```python
from build123d import *

# Parameters (mm, degrees)
SKETCH1_W           = 20
SKETCH1_H           = 14
SKETCH1_W_2         = 16
SKETCH1_H_2         = 10
BOSS_EXTRUDE1_DEPTH = 100
SKETCH2_W           = 50
SKETCH2_H           = 30
BOSS_EXTRUDE2_DEPTH = 2
SKETCH3_R           = 2.5
CUT_EXTRUDE1_DEPTH  = 2
SKETCH4_R           = 2.5
CUT_EXTRUDE2_DEPTH  = 106.399240984
FILLET1_R           = 1


with BuildPart() as part:
    # Sketch1 → Boss-Extrude1 (new body)
    with BuildSketch(Plane(origin=(0, 0, 0), x_dir=(1, 0, 0), z_dir=(0, 1, 0))):
        Rectangle(SKETCH1_W, SKETCH1_H)
        Rectangle(SKETCH1_W_2, SKETCH1_H_2, mode=Mode.SUBTRACT)
    extrude(amount=BOSS_EXTRUDE1_DEPTH)

    # Sketch2 → Boss-Extrude2 (add)
    with BuildSketch(Plane(origin=(0, 0, 0), x_dir=(-1, 0, 0), z_dir=(0, -1, 0))):
        Rectangle(SKETCH2_W, SKETCH2_H)
    extrude(amount=BOSS_EXTRUDE2_DEPTH)

    # Sketch3 → Cut-Extrude1 (cut)
    with BuildSketch(Plane(origin=(0, 0, 0), x_dir=(1, 0, 0), z_dir=(0, 1, 0))):
        with Locations(Location((18, -8, 0), (0, 0, 270))):
            Circle(SKETCH3_R)
        with Locations(Location((18, 8, 0), (0, 0, 90))):
            Circle(SKETCH3_R)
        with Locations(Location((-18, -8, 0), (0, 0, 90))):
            Circle(SKETCH3_R)
        with Locations(Location((-18, 8, 0), (0, 0, 270))):
            Circle(SKETCH3_R)
    extrude(amount=-CUT_EXTRUDE1_DEPTH, mode=Mode.SUBTRACT)

    # Sketch4 → Cut-Extrude2 (cut, through all)
    with BuildSketch(Plane.XY.offset(7)):
        with Locations((0, 87)):
            Circle(SKETCH4_R)
    extrude(amount=-CUT_EXTRUDE2_DEPTH, mode=Mode.SUBTRACT)

    # Fillet1
    fillet1_edges = [part.edges().sort_by_distance(p)[0] for p in [
        (-10, 100, 0),
        (0, 100, 7),
        (10, 100, 0),
        (0, 0, 7),
        (-10, 0, 0),
        (0, 0, -7),
        (10, 0, 0),
        (10, 50, 7),
        (-10, 50, 7),
        (-10, 50, -7),
        (10, 50, -7),
        (0, 100, -7),
    ]]
    fillet(fillet1_edges, radius=FILLET1_R)


solid = part.part
```
Model file for the job. Use its own axes, mm. A direction names the side the tool comes from. Give positions to 0.01 mm unless a question says otherwise; leave off trailing zeros. Order: outer loops, then holes, each group sorted by start corner. A loop starts at its lowest first (then second) coordinate and runs counter-clockwise, first axis right, second up.
1) Pin check, flat tips, straight feed: pin 1 (5 mm diameter, centred on y = 67.5, z = -2, fed in from +X); pin 2 (8 mm diameter, centred on y = 62.5, z = -0.5, fed in from -X); pin 3 (20 mm diameter, centred on x = -0.5, y = 67, fed in from +Z); pin 4 (4.5 mm diameter, centred on x = 18, z = -8, fed in from -Y). Stop position of each tip, or through.
2) Wall check: probe 1 along X at (y, z) = (-1.2, -8); probe 2 along X at (y, z) = (71, 1.75); probe 3 along Z at (x, y) = (-0.5, 38.5). Give the ranges that are in metal, low to high.
3) Saw through at B-B, the plane x = -18. Write the cut outline in (y, z).
4) 3-axis set-ups, long thin cutter, end or side, ignore diameter. For faces 1 (the flat face through (10, 49, 0)), 2 (the flat face through (0, -2, 0)), 3 (the flat face through (0, 0, -10)), 4 (the flat face through (0, 49, -7)): which of +Z, -Z, +X, -X, +Y, -Y reach the whole face in a straight line?
5) Saw through at C-C, the plane y = 36. Write the cut outline in (x, z).
6) Saw through at D-D, the plane z = -2.5. Write the cut outline in (x, y), then the cut area to 3 significant figures.
7) Mould opens along X. For faces 5 (the flat face through (-10, 49, 0)), 6 (the flat face through (0, -1, -15)), 7 (the cylindrical face through (20.11, -0.99, 9.34)), 8 (the flat face through (25, -1, 0)) say: +X half, -X half, draft (parallel to the pull), parting line (faces both ways), or undercut.
8) Saw through at A-A, the plane y = 87. Write the cut outline in (x, z), then the cut area to 3 significant figures.
Computed:
1. pin 1: stops at x = 10
1. pin 2: stops at x = -10
1. pin 3: stops at z = 7
1. pin 4: passes through
2. probe 1: x = -25 to -20.5, -15.5 to 15.5, 20.5 to 25
2. probe 2: x = -10 to -8, 8 to 10
2. probe 3: z = -7 to -5, 5 to 7
3. outline: (-2, -15) - (0, -15) - (0, -10.5) - (-2, -10.5) - close; (-2, -5.5) - (0, -5.5) - (0, 5.5) - (-2, 5.5) - close; (-2, 10.5) - (0, 10.5) - (0, 15) - (-2, 15) - close
4. face 1: +Z, -Z, +X, +Y
4. face 2: +Z, -Z, +X, -X, -Y
4. face 3: +Y
4. face 4: -Z, +X, -X, +Y
5. outline: (-10, -6) arc R1 ccw to (-9, -7) - (9, -7) arc R1 ccw to (10, -6) - (10, 6) arc R1 ccw to (9, 7) - (-9, 7) arc R1 ccw to (-10, 6) - close; hole (-8, -5) - (8, -5) - (8, 5) - (-8, 5) - close
6. outline: (-25, -2) - (25, -2) - (25, 0) - (11, 0) arc R1 cw to (10, 1) - (10, 99) arc R1 ccw to (9, 100) - (8, 100) - (8, 0) - (-8, 0) - (-8, 100) - (-9, 100) arc R1 ccw to (-10, 99) - (-10, 1) arc R1 cw to (-11, 0) - (-25, 0) - close
6. area: 500 mm2
7. face 5: -X half
7. face 6: draft
7. face 7: undercut
7. face 8: +X half
8. outline: (-10, -6) arc R1 ccw to (-9, -7) - (-2.5, -7) - (-2.5, -5) - (-8, -5) - (-8, 5) - (-2.5, 5) - (-2.5, 7) - (-9, 7) arc R1 ccw to (-10, 6) - close; (2.5, -7) - (9, -7) arc R1 ccw to (10, -6) - (10, 6) arc R1 ccw to (9, 7) - (2.5, 7) - (2.5, 5) - (8, 5) - (8, -5) - (2.5, -5) - close
8. area: 99.1 mm2
